Solid Edge part; units mm, degrees
sketch "Sketch1" plane through (0, 0, -15) normal (0, 0, 1) x (1, 0, 0)
  circle A0 centre (0, 21) radius 2.2
  line L0 (5, 26) -> (5, -5)
  line L1 (-5, -5) -> (5, -5)
  line L2 (-5, 26) -> (-5, -5)
  line L3 (-5, 26) -> (5, 26)
  circle A1 centre (0, 0) radius 2.2
extrude "ExtrudedProtrusion_1" add sketch "Sketch1" against normal blind 10
properties material "ABS Plastic, medium impact"
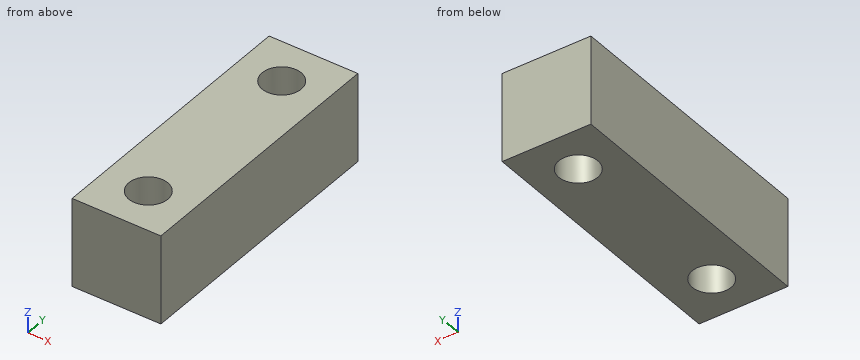
For this review, take the finished solid that the model builds, in its own axes (mm). Round coordinates to 2 decimals unless told otherwise and drop trailing zeros. Write each loop counter-clockwise with the first axis right and the second up, starting at its lowest first coordinate (ties: lowest second). Pieces come first, ordered by that corner, then holes. Notation, with made-up numbers: (77.5, 31.5) -> (87.5, 31.5) arc R22 ccw to (87.5, 66.5) -> close; hole circle Ø3 at (69, 20.5). An arc over 180 degrees is marked (long way). One line per question, with ' | ' between items. Start each with the question number.
1) Add section A-A (x = 0). Write out the cut boundary in (y, z), and give its area (3 significant figures).
2) Wall thickness on line 1 along Y through (x, z) = (0, -20.25); line 2 along Y through (x, z) = (-1.25, -21.75); line 3 along X through (y, z) = (20, -23): over which ranges is each line inside the solid? List them lowest first.
3) Add section B-B (y = 21). Write out the cut boundary in (x, z).
4) Add section C-C (z = -21.25). Write out the cut boundary in (x, y).
Reported:
1) outline: (-5, -25) -> (-2.2, -25) -> (-2.2, -15) -> (-5, -15) -> close; (2.2, -25) -> (18.8, -25) -> (18.8, -15) -> (2.2, -15) -> close; (23.2, -25) -> (26, -25) -> (26, -15) -> (23.2, -15) -> close | area: 222 mm²
2) line 1: y = -5 to -2.2, 2.2 to 18.8, 23.2 to 26 | line 2: y = -5 to -1.81, 1.81 to 19.19, 22.81 to 26 | line 3: x = -5 to -1.96, 1.96 to 5
3) outline: (-5, -25) -> (-2.2, -25) -> (-2.2, -15) -> (-5, -15) -> close; (2.2, -25) -> (5, -25) -> (5, -15) -> (2.2, -15) -> close
4) outline: (-5, -5) -> (5, -5) -> (5, 26) -> (-5, 26) -> close; hole circle Ø4.4 at (0, 0); hole circle Ø4.4 at (0, 21)
